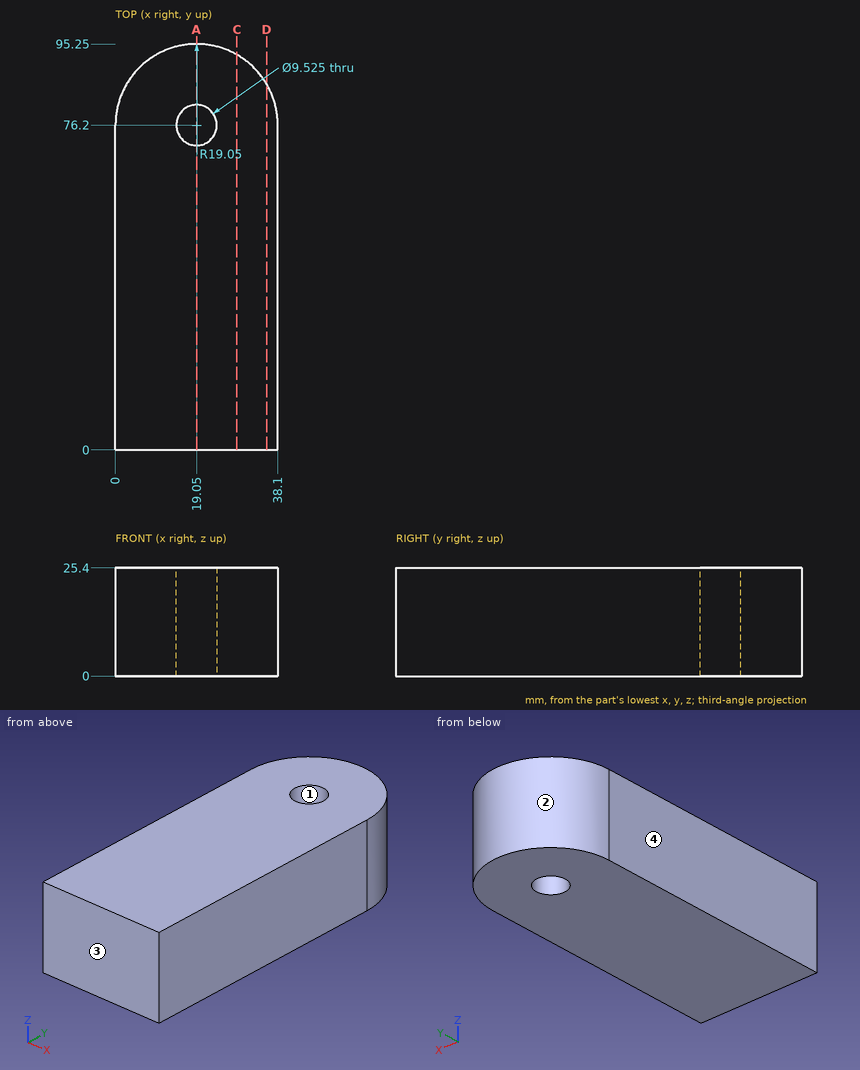
Geometry: see drawing. Coordinates: mm, zero at the bounding-box minimum. Give positions to 0.01 mm unless a question says otherwise; leave off trailing zeros. Order: outer loops, then holes, each group sorted by start corner. A loop starts at its lowest first (then second) coordinate and runs counter-clockwise, first axis right, second up.
Q1. Draft query along X for the marked faces 1, 2, 3 and 4. Return one class per face: +X half, -X half, draft (parallel to the pull), parting line (faces both ways), or undercut.
Checked values:
face 1: undercut
face 2: parting line
face 3: draft
face 4: -X half
Q2. Ray query, probe 1 along Y at (x, z) = (19.05, 6.5); probe 2 along X at (y, z) = (72.5, 24.75); probe 3 along X at (y, z) = (73, 10.75). Return the intervals inside material, ascending.
Checked values:
probe 1: y = 0 to 71.44, 80.96 to 95.25
probe 2: x = 0 to 16.05, 22.05 to 38.1
probe 3: x = 0 to 15.52, 22.58 to 38.1
Q3. Section D-D on x = 35.5. Output: boundary loops of the cut face in (y, z).
Checked values:
outline: (0, 0) - (85.81, 0) - (85.81, 25.4) - (0, 25.4) - close
Q4. Contact query for flat-ended pins moving along their axis: pin 1 Ø6 at (x, z) = (32.5, 3.5) entering from +Y; pin 2 Ø5 at (x, z) = (18.5, 15) entering from +Y; pin 3 Ø7.5 at (x, y) = (19.05, 76.2) entering from +Z. Output: stop coordinate, or through.
Checked values:
pin 1: stops at y = 92.13
pin 2: stops at y = 95.25
pin 3: passes through
Q5. Section A-A on x = 19.05. Output: boundary loops of the cut face in (y, z), and give its area (3 significant figures).
Checked values:
outline: (0, 0) - (71.44, 0) - (71.44, 25.4) - (0, 25.4) - close; (80.96, 0) - (95.25, 0) - (95.25, 25.4) - (80.96, 25.4) - close
area: 2,180 mm2
Q6. Section C-C on x = 28.5. Output: boundary loops of the cut face in (y, z), and give its area (3 significant figures).
Checked values:
outline: (0, 0) - (92.74, 0) - (92.74, 25.4) - (0, 25.4) - close
area: 2,360 mm2
